Geometry check sheet. Reference: the model listing, model coordinates, mm. Coordinates: 2 decimals unless noted, no trailing zeros. Write each loop counter-clockwise with the first axis right and the second up, starting at its lowest first coordinate (ties: lowest second). Pieces come first, ordered by that corner, then holes. Notation, with made-up numbers: (88, 63) -> (99, 63) arc R12 cw to (99, 83) -> close; hole circle Ø7 at (-6.75, -2.5). An arc over 180 degrees is marked (long way). One line per question, with ' | ' between items.
```python
from build123d import *

# Parameters (mm, degrees)
SKETCH1_R           = 25
SKETCH1_R_2         = 22
BOSS_EXTRUDE1_DEPTH = 600


# Read off the part's stored shape, not the designer's step: Cut-Revolve3
with BuildPart() as part:
    # Sketch1 → Boss-Extrude1 (new body)
    with BuildSketch(Plane(origin=(0, 0, 0), x_dir=(1, 0, 0), z_dir=(0, 1, 0))):
        with Locations(Location((0, 0, 0), (0, 0, 270))):
            Circle(SKETCH1_R)
        with Locations(Location((0, 0, 0), (0, 0, 270))):
            Circle(SKETCH1_R_2, mode=Mode.SUBTRACT)
    extrude(amount=BOSS_EXTRUDE1_DEPTH)

    # Cut-Revolve3 outline → Cut-Revolve3 (revolve, cut)
    with BuildSketch(Plane(origin=(-6.639528096, 380, 0), x_dir=(1, 0, 0), z_dir=(0, -1, 0))):
        Polygon((0, -25.000000429), (6.639528344, -25.000000429), (3.482816484, -19.532415103), (0, -19.532415103), align=None)
    cut_revolve3 = revolve(axis=Axis((-6.639528096, 380, 0), (0, 0, 1)), mode=Mode.SUBTRACT)

    # Sketch5 → Cut-Revolve4 (revolve, cut)
    with BuildSketch(Plane(origin=(-103.136389545, 110, -329.994936254), x_dir=(-1, 0, 0), z_dir=(0, -1, 0)), mode=Mode.PRIVATE) as cut_revolve4_sk:
        Polygon((-103.136389545, -304.994936254), (-103.136389545, -316.494936254), (-96.496861449, -304.994936254), align=None)
    cut_revolve4 = revolve(cut_revolve4_sk.sketch.rotate(Axis((0, 110, -25), (0, 0, 1)), 31.719951759), axis=Axis((0, 110, -25), (0, 0, 1)), mode=Mode.SUBTRACT)

    # Mirror3: Cut-Revolve3, Cut-Revolve4 across plane
    add(cut_revolve3.mirror(Plane.XY), mode=Mode.SUBTRACT)
    add(cut_revolve4.mirror(Plane.XY), mode=Mode.SUBTRACT)


solid = part.part
```
(1) Draft check along Y on faces 1 (the face through (-22.1, 0, 1.7)), 2 (the face through (-21.477, 295.8, -4.769)), 3 (the face through (-4.69, 109.24, 21.73)), 4 (the face through (-22.1, 600, 1.7)). Enter one of: pulls with the +Y half, pulls with the -Y half, needs draft (parallel to the pull), parting line crosses it, or undercut.
Answers below:
face 1: pulls with the -Y half | face 2: needs draft | face 3: undercut | face 4: pulls with the +Y half
(2) Cross-section at C-C (y = 157). Record the cut outline in (x, z).
Answers below:
outline: circle Ø50 at (0, 0); hole circle Ø44 at (0, 0)
(3) Material ranges on line 1 (Y direction, x = -2.5, z = -22); line 2 (X direction, y = 202, z = 0); line 3 (Z direction, x = -1, y = 421.5), recorded low to high.
Answers below:
line 1: y = 0 to 105.78, 114.22 to 377.36, 382.64 to 600 | line 2: x = -25 to -22, 22 to 25 | line 3: z = -24.98 to -21.98, 21.98 to 24.98
(4) Depth check by flat-ended pin: P1, Ø6, axis at y = 477.5, z = -3, coming from the +X side; P2, Ø1.5, axis at x = 8, y = 305.5, coming from the -Z side; P3, Ø10, axis at x = 8.5, y = 445.5, coming from the -Z side. Enter the tip coordinate at first touch or a pass-through.
Answers below:
P1: stops at x = 25 | P2: stops at z = -23.93 | P3: stops at z = -24.75
(5) Cross-section at A-A (z = 0). Record the cut outline in (x, y).
Answers below:
outline: (-25, 0) -> (-22, 0) -> (-22, 600) -> (-25, 600) -> close; (22, 0) -> (25, 0) -> (25, 600) -> (22, 600) -> close
(6) Cross-section at B-B (y = 380). Record the cut outline in (x, z).
Answers below:
outline: (-11.62, -22.13) -> (-10.12, -19.53) arc R22 cw to (-10.12, 19.53) -> (-11.62, 22.13) arc R25 ccw to start; (-1.77, -21.93) -> (0, -25) arc R25 ccw to (0, 25) -> (-1.77, 21.93) arc R22 cw (long way) to start
